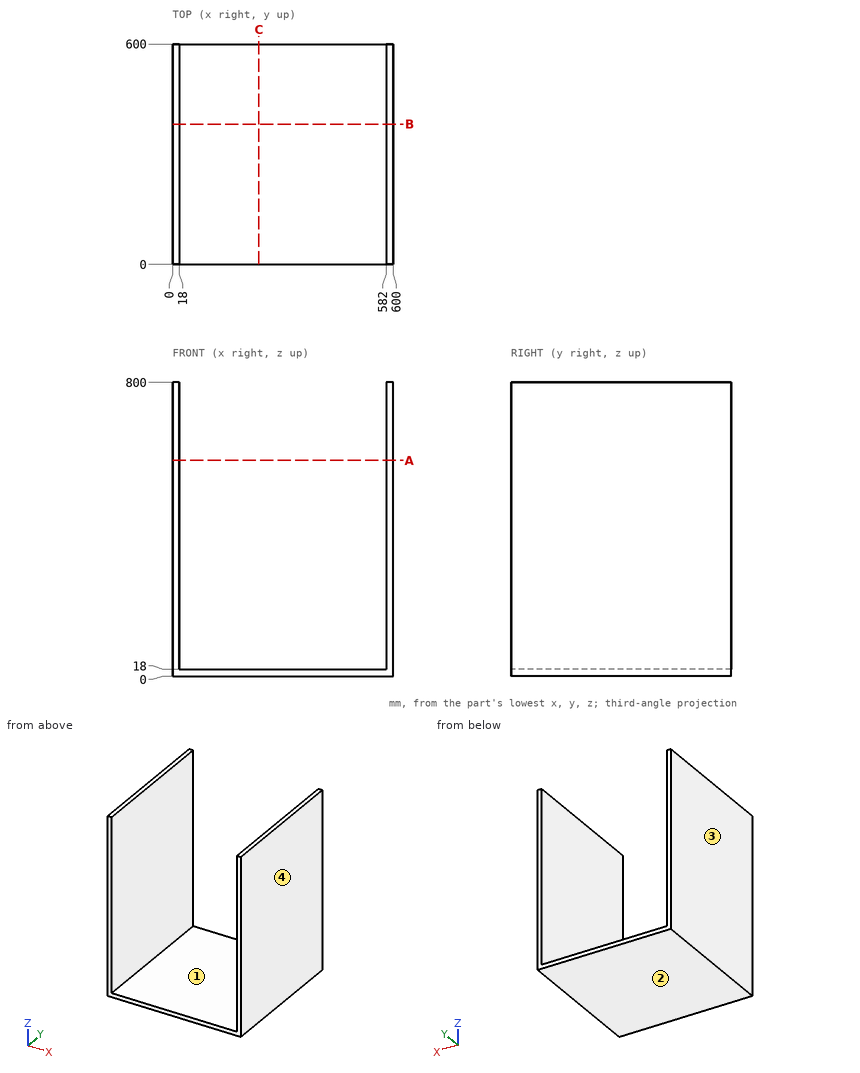
Verification items for this drawing (mm, ordinates from the low corner). Round coordinates to 2 decimals unless told otherwise and drop trailing zeros. Order: outer loops, then holes, each group sorted by start corner. A loop starts at its lowest first (then second) coordinate and runs counter-clockwise, first axis right, second up. Notation, with made-up numbers: M 23.5,16.25 L 70.5,16.25 A26 cw 70.5,53.25 Z; hole C 70,85.25 d9. An arc over 180 degrees is marked long. Answer in a Markdown table with one row per item. Add a question column.
Item 1: Draft check along X on the marked faces 1, 2, 3 and 4. Enter one of: released by +X, released by -X, zero draft, split by the parting line, or undercut.
Item 2: Depth check by flat-ended pin: pin 1 Ø5 at (x, y) = (276, 471.5) entering from +Z. Enter the tip coordinate at first touch or a pass-through.
Item 3: Sectioned sample at C-C, the plane x = 235. Enter the section's corners in (y, z), plus the area to 3 significant figures.
Item 4: Sectioned sample at B-B, the plane y = 381.5. Enter the section's corners in (x, z).
Item 5: Sectioned sample at A-A, the plane z = 587. Enter the section's corners in (x, y).
Item 6: Material ranges on L1, parallel to X at y = 119, z = 255.5; L2, parallel to Z at x = 429, y = 44, recorded low to high. Write a range as [from, to].
Filled in:
| question | item | result |
|---|---|---|
| 1 | face 1 | undercut |
| 1 | face 2 | zero draft |
| 1 | face 3 | released by -X |
| 1 | face 4 | released by +X |
| 2 | pin 1 | stops at z = 18 |
| 3 | outline | M 0,0 L 600,0 L 600,18 L 0,18 Z |
| 3 | area | 10,800 mm² |
| 4 | outline | M 0,0 L 600,0 L 600,800 L 582,800 L 582,18 L 18,18 L 18,800 L 0,800 Z |
| 5 | outline | M 0,0 L 18,0 L 18,600 L 0,600 Z; M 582,0 L 600,0 L 600,600 L 582,600 Z |
| 6 | L1 | x = [0, 18], [582, 600] |
| 6 | L2 | z = [0, 18] |
